Read the model definition and answer for the solid it produces. Units are mm, in the model's axes. A direction names the side the tool comes from. Coordinates: 2 decimals unless noted, no trailing zeros. Order: outer loops, then holes, each group sorted by start corner. A loop starts at its lowest first (then second) coordinate and runs counter-clockwise, first axis right, second up. Notation, with made-up numbers: (47, -26) - (64, -26) arc R20 cw to (64, 8) - close; hole circle Ø7 at (24, 36.25). An arc over 180 degrees is marked (long way). Use one line per item in the form item = value.
```python
from build123d import *

# Parameters (mm, degrees)
F1_DEPTH = 6.35
F3_DEPTH = 6.35
F2_R     = 12.7
F4_DEPTH = 12.7
F5_R     = 6.35
F6_DEPTH = 19.05


with BuildPart() as f1:
    # F0 (on Top) → F1 (new body)
    with BuildSketch(Plane.XY):
        Polygon((0, 25.4), (0, 0), (19.05, 0), (31.75, 12.7), (31.75, 25.4), align=None)
    extrude(amount=-F1_DEPTH)

    # F2 (on face) → F3 (join)
    with BuildSketch(Plane.XY):
        with BuildLine():
            Line((0, 0), (0, 25.4))
            ThreePointArc((0, 25.4), (-12.7, 12.7), (0, 0))
        make_face()
    extrude(amount=-F3_DEPTH)

    # F2 (on face) → F4 (join)
    with BuildSketch(Plane.XY):
        with Locations((0, 12.7)):
            Circle(F2_R)
    extrude(amount=F4_DEPTH)

    # F5 (on face) → F6 (cut)
    with BuildSketch(Plane.XY.offset(12.7)):
        with Locations((0, 12.7)):
            Circle(F5_R)
    extrude(amount=-F6_DEPTH, mode=Mode.SUBTRACT)


solid = f1.part
```
(1) Straight lines are drawn through the part: L1, parallel to Y at x = 0, z = 2.5; L2, parallel to Z at x = 19, y = 14.5; L3, parallel to Y at x = -5.5, z = 2. For each, find the intervals that lie inside material, in ascending order.
Answer list:
L1 = 0 to 6.35, 19.05 to 25.4
L2 = -6.35 to 0
L3 = 1.25 to 9.53, 15.87 to 24.15
(2) Which of the six approach directions +Z, -Z, +X, -X, +Y, -Y give full straight-line access (tool end or side, diameter ignored) to faces 1 (the flat face through (9, 13, -6.35)), 2 (the cylindrical face through (-12.688, 13.258, 5.158))?
Answer list:
face_1 = -Z, +X, -X, +Y, -Y
face_2 = +Z
(3) Section D-D, the plane y = 16.25 is taken. Write down the section's boundary in (x, z).
Answer list:
outline = (-12.19, -6.35) - (-5.26, -6.35) - (-5.26, 12.7) - (-12.19, 12.7) - close; (5.26, -6.35) - (31.75, -6.35) - (31.75, 0) - (12.19, 0) - (12.19, 12.7) - (5.26, 12.7) - close
(4) Section B-B, the plane y = 10.5 is taken. Write down the section's boundary in (x, z).
Answer list:
outline = (-12.51, -6.35) - (-5.96, -6.35) - (-5.96, 12.7) - (-12.51, 12.7) - close; (5.96, -6.35) - (29.55, -6.35) - (29.55, 0) - (12.51, 0) - (12.51, 12.7) - (5.96, 12.7) - close
(5) Section A-A, the plane x = -5 is taken. Write down the section's boundary in (y, z), then the cut area to 3 significant figures.
Answer list:
outline = (1.03, -6.35) - (8.79, -6.35) - (8.79, 12.7) - (1.03, 12.7) - close; (16.61, -6.35) - (24.37, -6.35) - (24.37, 12.7) - (16.61, 12.7) - close
area = 296 mm2
(6) Given pin 1 Ø2 at (y, z) = (15, -3) entering from -X; pin 2 Ø2 at (x, z) = (-1.5, 6.5) entering from -Y; pin 3 Ø8 at (y, z) = (8.5, 4.5) entering from -X, each flat-ended and moving along its own axis, determine where each tip first touches the part or whether it passes through.
Answer list:
pin_1 = -12.63
pin_2 = 0.01
pin_3 = -12.7
(7) The mould has two halves that part along X. Classify faces 3 (the flat face through (31.75, 19, -3)), 4 (the cylindrical face through (3.414, 18.054, 3.308)), 5 (the flat face through (19, 13, 0)): +X half, -X half, draft (parallel to the pull), parting line (faces both ways), or undercut.
Answer list:
face_3 = +X half
face_4 = undercut
face_5 = draft
(8) Section C-C, the plane z = -0.75 is taken. Write down the section's boundary in (x, y).
Answer list:
outline = (0, 0) - (19.05, 0) - (31.75, 12.7) - (31.75, 25.4) - (0, 25.4) arc R12.7 ccw to start; hole circle Ø12.7 at (0, 12.7)
